from build123d import *

# Parameters (mm, degrees)
F0_R     = 4
F0_R_2   = 11
F1_DEPTH = 3.5
F2_SIZE  = 0.5
F3_R     = 5


with BuildPart() as f1:
    # F0 (on Top) → F1 (new body, symmetric)
    with BuildSketch(Plane.XY):
        with BuildLine():
            ThreePointArc((-11.25833, 6.5), (0, 13), (11.25833, 6.5))
            Line((11.25833, 6.5), (10, 35))
            Line((10, 35), (-10, 35))
            Line((-10, 35), (-11.25833, 6.5))
        make_face()
        with Locations((-5, 30)):
            Circle(F0_R, mode=Mode.SUBTRACT)
        with Locations((5, 30)):
            Circle(F0_R, mode=Mode.SUBTRACT)
        with BuildLine():
            ThreePointArc((0, -13), (9.192388, -9.192388), (13, 0))
            ThreePointArc((13, 0), (12.557036, 3.364648), (11.25833, 6.5))
            ThreePointArc((11.25833, 6.5), (0, 13), (-11.25833, 6.5))
            ThreePointArc((-11.25833, 6.5), (-11.25833, -6.5), (0, -13))
        make_face()
        Circle(F0_R_2, mode=Mode.SUBTRACT)
        with BuildLine():
            Line((-25.310889, -26.160254), (0, -13))
            ThreePointArc((0, -13), (-11.25833, -6.5), (-11.25833, 6.5))
            Line((-11.25833, 6.5), (-35.310889, -8.839746))
            Line((-35.310889, -8.839746), (-25.310889, -26.160254))
        make_face()
        with Locations((-23.480762, -19.330127)):
            Circle(F0_R, mode=Mode.SUBTRACT)
        with Locations((-28.480762, -10.669873)):
            Circle(F0_R, mode=Mode.SUBTRACT)
        with BuildLine():
            ThreePointArc((11.25833, 6.5), (12.557036, 3.364648), (13, 0))
            ThreePointArc((13, 0), (9.192388, -9.192388), (0, -13))
            Line((0, -13), (25.310889, -26.160254))
            Line((25.310889, -26.160254), (35.310889, -8.839746))
            Line((35.310889, -8.839746), (11.25833, 6.5))
        make_face()
        with Locations((23.480762, -19.330127)):
            Circle(F0_R, mode=Mode.SUBTRACT)
        with Locations((28.480762, -10.669873)):
            Circle(F0_R, mode=Mode.SUBTRACT)
    extrude(amount=F1_DEPTH, both=True)

    # F2
    f2_edges = [f1.edges().sort_by_distance(p)[0] for p in [
        (-9, 30, 3.5),
        (1, 30, 3.5),
        (-11, 0, 3.5),
        (-32.480762, -10.669873, 3.5),
        (-27.480762, -19.330127, 3.5),
        (24.480762, -10.669873, 3.5),
        (19.480762, -19.330127, 3.5),
        (-11, 0, -3.5),
        (-27.480762, -19.330127, -3.5),
        (-32.480762, -10.669873, -3.5),
        (19.480762, -19.330127, -3.5),
        (24.480762, -10.669873, -3.5),
        (1, 30, -3.5),
        (-9, 30, -3.5),
    ]]
    chamfer(f2_edges, length=F2_SIZE)

    # F3
    f3_edges = [f1.edges().sort_by_distance(p)[0] for p in [
        (-25.310889, -26.160254, 0),
        (-35.310889, -8.839746, 0),
        (25.310889, -26.160254, 0),
        (35.310889, -8.839746, 0),
        (10, 35, 0),
        (-10, 35, 0),
        (-11.25833, 6.5, 0),
        (11.25833, 6.5, 0),
        (0, -13, 0),
    ]]
    fillet(f3_edges, radius=F3_R)


solid = f1.part
The listing builds one solid part. Answer for the finished solid, in the listing's coordinates (mm). Coordinates: 2 decimals unless noted, no trailing zeros. Write each loop counter-clockwise with the first axis right and the second up, starting at its lowest first coordinate (ties: lowest second). Pieces come first, ordered by that corner, then holes. Notation, with made-up numbers: M 38.5,82.5 L 73.5,82.5 A22 cw 73.5,101.5 Z; hole C 85,-37 d9. An arc over 180 degrees is marked long. Put each result on its own line as item: value. Start each with the question number.
1. Consider line 1 (Y direction, x = -2, z = -3); line 2 (Y direction, x = 7.5, z = -2.5); line 3 (X direction, y = -10, z = -0.75). Determine where each line is inside the solid, lowest interval first. Write a range as from..to.
2. A flat-ended cylindrical pin translates along its axis: P1, Ø4, axis at y = 18.5, z = 0, coming from the +X side. Find the tip coordinate at first contact, or state that the pin passes through.
3. A cutting plane is placed at B-B on y = 15. Write down the section's boundary in (x, z), then the cut area to 3 significant figures.
4. A cutting plane is placed at A-A on z = -2.25. Write down the section's boundary in (x, y).
5. A cutting plane is placed at C-C on x = 15.5. Write down the section's boundary in (y, z), then the cut area to 3 significant figures.
6. For a pull along X with two mould halves and no side action, classify faces 1 (the cylindrical face through (-0.034, -13.636, 0.049)), 2 (the cylindrical face through (8.634, 33.649, -0.049)), 3 (the flat face through (-3, 12, -3.5)) as pulls with the +X half, pulls with the -X half, needs draft (parallel to the pull), parting line crosses it, or undercut.
Resolved:
1. line 1: y = -14.05..-10.82, 10.82..27.35, 32.65..35
1. line 2: y = -16.9..-8.05, 8.05..26.88, 33.12..34.45
1. line 3: x = -33.57..-32.42, -24.54..-4.58, 4.58..24.54, 32.42..33.57
2. P1: stops at x = 10.82
3. outline: M -10.88,-3.5 L 10.88,-3.5 L 10.88,3.5 L -10.88,3.5 Z
3. area: 152 mm2
4. outline: M -32.92,-12.98 L -27.7,-22.02 A5 ccw -21.07,-23.95 L -2.31,-14.2 A5 cw 2.31,-14.2 L 21.07,-23.95 A5 ccw 27.7,-22.02 L 32.92,-12.98 A5 ccw 31.28,-6.27 L 13.45,5.1 A5 cw 11.14,9.1 L 10.21,30.22 A5 ccw 5.22,35 L -5.22,35 A5 ccw -10.21,30.22 L -11.14,9.1 A5 cw -13.45,5.1 L -31.28,-6.27 A5 ccw Z; hole C -28.48,-10.67 d8; hole C -23.48,-19.33 d8; hole C 0,0 d22; hole C -5,30 d8; hole C 5,30 d8; hole C 23.48,-19.33 d8; hole C 28.48,-10.67 d8
5. outline: M -21.06,-3.5 L 3.79,-3.5 L 3.79,3.5 L -21.06,3.5 Z
5. area: 174 mm2
6. face 1: undercut
6. face 2: pulls with the +X half
6. face 3: needs draft
